from build123d import *

# Parameters (mm, degrees)
F1_DEPTH = 50
F2_R     = 3
F3_W     = 40
F3_H     = 40
F4_DEPTH = 2


with BuildPart() as f1:
    # F0 (on Front) → F1 (new body)
    with BuildSketch(Plane.XZ):
        Polygon((0, 9), (0, 6), (2, 6), (4, 9), align=None)
        Polygon((2, 6), (0, 6), (0, 0), (12, 0), (12, 2), (6, 2), (6, 4), (56, 4), (58, 3.95681), (58, 6), (56, 6), align=None)
        Polygon((54, 9), (56, 6), (58, 6), (58, 9), align=None)
    extrude(amount=F1_DEPTH)

    # F2
    f2_edges = [f1.edges().sort_by_distance(p)[0] for p in [
        (0, -25, 9),
        (58, -25, 9),
    ]]
    fillet(f2_edges, radius=F2_R)

    # F3 (on face) → F4 (cut)
    with BuildSketch(Plane.XY.offset(6)):
        with Locations((29, -25)):
            Rectangle(F3_W, F3_H)
    extrude(amount=-F4_DEPTH, mode=Mode.SUBTRACT)


solid = f1.part
Work out the finished part from the listing and answer in its coordinate system (mm). A direction names the side the tool comes from. Give positions to 0.01 mm unless a question says otherwise; leave off trailing zeros. Loops run counter-clockwise (first coordinate to the right, second up) from the corner with the lowest first, then second, coordinate; pieces in that order, holes last. Notation, with made-up numbers: (5.5, 70) - (27.5, 70) arc R17 ccw to (27.5, 98) - close; hole circle Ø2 at (21, 10). An arc over 180 degrees is marked (long way). Answer in a Markdown table with one row per item. Add a question column.
Q1. Each of these flat-tipped pins is pushed along its axis until it touches: P1, Ø2, axis at x = 11, y = -40, coming from the -Z side; P2, Ø4, axis at y = -35, z = 1, coming from the +X side; P3, Ø1.8, axis at x = 8, y = -23, coming from the +Z side; P4, Ø0.6, axis at y = -29.5, z = 3, coming from the +X side. Where does it stop, or does it pass through?
Q2. Consider line 1 along X through (y, z) = (-31, 4.25); line 2 along X through (y, z) = (-35, 0.5); line 3 along Z through (x, y) = (54.5, -38). Determine where each line is inside the solid, lowest interval first.
Q3. The part is cut by section D-D (z = 8). Determine the outline of the cut face in (x, y), and give its area (3 significant figures).
Q4. A tool of negligible diameter and unlimited length cuts with its end or side. For faces 1 (the flat face through (12, -25, 1)), 2 (the flat face through (9, -25, 5)), 3 (the flat face through (49, -25, 5)), 4 (the flat face through (55, -24.6, 7.5)), from which of +Z, -Z, +X, -X, +Y, -Y can it reach the whole face along a straight path? Write none if from no direction.
Q5. The part is cut by section C-C (z = 5). Determine the outline of the cut face in (x, y).
Q6. The part is cut by section B-B (x = 33). Determine the outline of the cut face in (y, z), and give its area (3 significant figures).
Q7. The part is cut by section A-A (y = -16). Determine the outline of the cut face in (x, z).
Q8. Determine the mould class of faces 5 (the flat face through (29, -47, 6)), 6 (the flat face through (22.4, -50, 4.2)), 7 (the flat face through (29, -45, 5)), 8 (the flat face through (22.4, 0, 4.2)) for opening direction Y: released by +Y, released by -Y, zero draft, split by the parting line, or undercut.
Solution:
| question | item | result |
|---|---|---|
| 1 | P1 | stops at z = 0 |
| 1 | P2 | stops at x = 12 |
| 1 | P3 | stops at z = 6 |
| 1 | P4 | stops at x = 6 |
| 2 | line 1 | x = 0 to 9, 49 to 58 |
| 2 | line 2 | x = 0 to 12 |
| 2 | line 3 | z = 4 to 6, 8.25 to 9 |
| 3 | outline | (0.76, -50) - (3.33, -50) - (3.33, 0) - (0.76, 0) - close; (54.67, -50) - (57.24, -50) - (57.24, 0) - (54.67, 0) - close |
| 3 | area | 257 mm² |
| 4 | face 1 | -Z, +X, +Y, -Y |
| 4 | face 2 | +Z |
| 4 | face 3 | +Z, -Z |
| 4 | face 4 | +Y, -Y |
| 5 | outline | (0, -50) - (58, -50) - (58, 0) - (0, 0) - close; hole (9, -45) - (49, -45) - (49, -5) - (9, -5) - close |
| 6 | outline | (-50, 4) - (-45, 4) - (-45, 6) - (-50, 6) - close; (-5, 4) - (0, 4) - (0, 6) - (-5, 6) - close |
| 6 | area | 20.0 mm² |
| 7 | outline | (0, 0) - (12, 0) - (12, 2) - (6, 2) - (6, 4) - (9, 4) - (9, 6) - (2, 6) - (4, 9) - (3, 9) arc R3 ccw to (0, 6) - close; (49, 4) - (56, 4) - (58, 3.96) - (58, 6) arc R3 ccw to (55, 9) - (54, 9) - (56, 6) - (49, 6) - close |
| 8 | face 5 | zero draft |
| 8 | face 6 | released by -Y |
| 8 | face 7 | undercut |
| 8 | face 8 | released by +Y |
